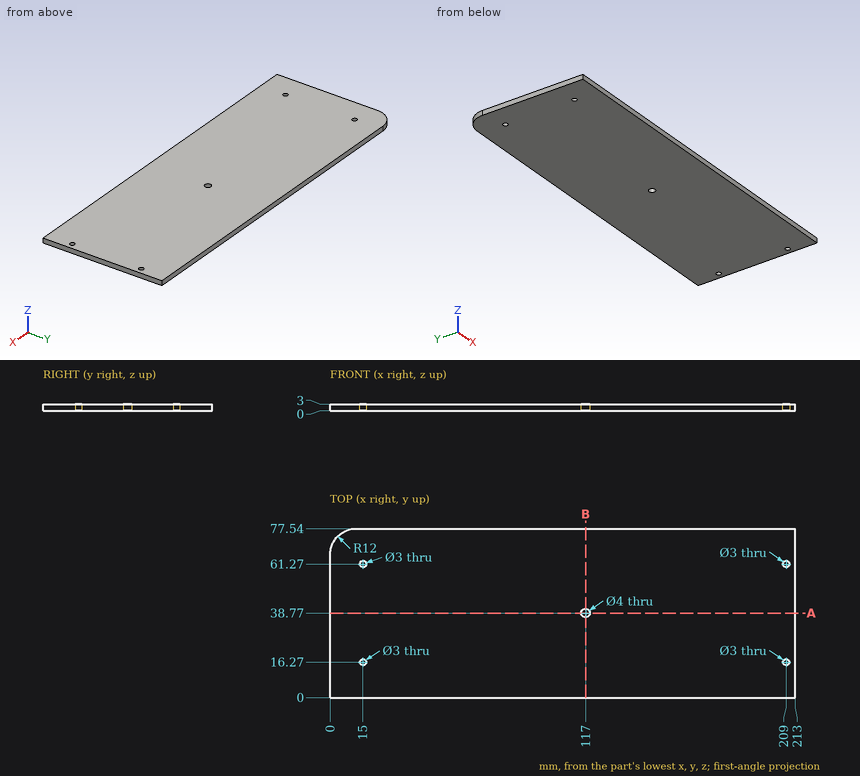
Geometry check sheet. Reference: drawing and pictorial views, mm from the part's lowest x, y, z. Round coordinates to 2 decimals unless told otherwise and drop trailing zeros. Loops run counter-clockwise (first coordinate to the right, second up) from the corner with the lowest first, then second, coordinate; pieces in that order, holes last. Notation, with made-up numbers: (-26.75, 78.25) -> (24.25, 78.25) arc R22 ccw to (24.25, 101.25) -> close; hole circle Ø6 at (55.25, -21). An arc over 180 degrees is marked (long way). Use a Markdown table: item, result.
(1) Sectioned sample at A-A (y = 38.77). Enter the section's corners in (x, z).
Calculated:
| item | result |
|---|---|
| outline | (0, 0) -> (115, 0) -> (115, 3) -> (0, 3) -> close; (119, 0) -> (213, 0) -> (213, 3) -> (119, 3) -> close |
(2) Sectioned sample at B-B (x = 117). Enter the section's corners in (y, z).
Calculated:
| item | result |
|---|---|
| outline | (0, 0) -> (36.77, 0) -> (36.77, 3) -> (0, 3) -> close; (40.77, 0) -> (77.54, 0) -> (77.54, 3) -> (40.77, 3) -> close |
(3) Scan lines: probe 1 along Y at (x, z) = (209, 1.1); probe 2 along X at (y, z) = (62.5, 1.2); probe 3 along X at (y, z) = (71.5, 2.9). Record each from-to range of solid material in increasing order.
Calculated:
| item | result |
|---|---|
| probe 1 | 0 to 14.77, 17.77 to 59.77, 62.77 to 77.54 |
| probe 2 | 0 to 14.14, 15.86 to 208.14, 209.86 to 213 |
| probe 3 | 1.58 to 213 |
(4) Go/stop test with a flat-tipped pin: P1, Ø4, axis at x = 209, y = 16.27, coming from the +Z side. Record where the tip stops, or that it passes through.
Calculated:
| item | result |
|---|---|
| P1 | z = 3 |
